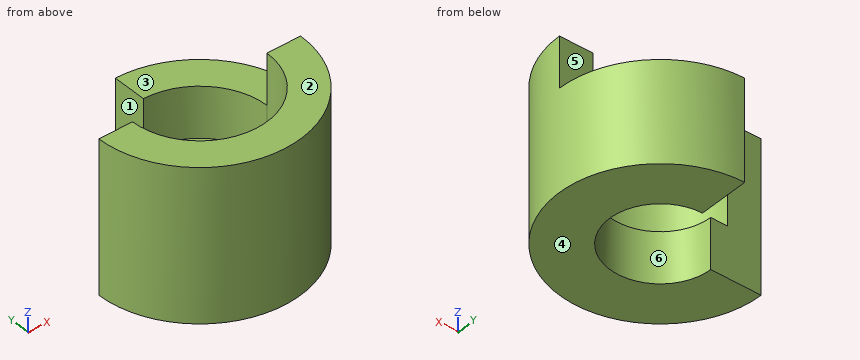
```python
from build123d import *

# Parameters (mm, degrees)
BOSS_EXTRUDE1_DEPTH = 9
SKETCH2_W           = 6
SKETCH2_H           = 6
CUT_EXTRUDE1_DEPTH  = 3
SKETCH3_R           = 4
CUT_EXTRUDE2_DEPTH  = 6


with BuildPart() as part:
    # Sketch1 → Boss-Extrude1 (new body)
    with BuildSketch(Plane.XY):
        with BuildLine():
            Line((-6, 0), (-3, 0))
            ThreePointArc((-3, 0), (2.121320344, -2.121320344), (0, 3))
            Line((0, 3), (0, 6))
            ThreePointArc((0, 6), (4.242640687, -4.242640687), (-6, 0))
        make_face()
    extrude(amount=BOSS_EXTRUDE1_DEPTH)

    # Sketch2 → Cut-Extrude1 (cut)
    with BuildSketch(Plane.XY.offset(9)):
        with Locations((3, 3)):
            Rectangle(SKETCH2_W, SKETCH2_H)
    extrude(amount=-CUT_EXTRUDE1_DEPTH, mode=Mode.SUBTRACT)

    # Sketch3 → Cut-Extrude2 (cut)
    with BuildSketch(Plane.XY.offset(9)):
        Circle(SKETCH3_R)
    extrude(amount=-CUT_EXTRUDE2_DEPTH, mode=Mode.SUBTRACT)


solid = part.part
```
Work out the finished part from the listing and answer in its coordinate system (mm). Face numbers are marked on the shaded views. A direction names the side the tool comes from. Give positions to 0.01 mm unless a question says otherwise; leave off trailing zeros. Loops run counter-clockwise (first coordinate to the right, second up) from the corner with the lowest first, then second, coordinate; pieces in that order, holes last. Notation, with made-up numbers: (83.25, -22.5) -> (135.25, -22.5) arc R32 cw to (135.25, 14.5) -> close; hole circle Ø9 at (-35, 26). An arc over 180 degrees is marked (long way). Write item = value, one per line. Start each with the question number.
(1) Which of the six approach directions +Z, -Z, +X, -X, +Y, -Y give full straight-line access (tool end or side, diameter ignored) to the marked faces 1, 2 and 3?
(2) Find section B-B on z = 5. Give the vertices of the cut face in (x, y), and give its area (3 significant figures).
(3) Find section A-A on y = -0.5. Give the vertices of the cut face in (x, z).
(4) Find section C-C on x = -1.5. Give the vertices of the cut face in (y, z), and give its area (3 significant figures).
(5) Find the intervals of material crossed by probe 1 along Z at (x, y) = (3.75, -0.5); probe 2 along X at (y, z) = (-2.75, 6.75); probe 3 along Z at (x, y) = (4, 1.5), in increasing order. Write a range as from..to.
(6) Given pin 1 Ø3.5 at (y, z) = (5, 4) entering from -X; pin 2 Ø1.8 at (x, y) = (1.5, 3.5) entering from +Z; pin 3 Ø1 at (x, z) = (4.5, 7.5) entering from +Y, each flat-ended and moving along its own axis, determine where each tip first touches the part or whether it passes through.
(7) The mould has two halves that part along Y. Classify the marked faces 4, 5 and 6: +Y half, -Y half, draft (parallel to the pull), parting line (faces both ways), or undercut.
(8) Find section D-D on y = -3.5. Give the vertices of the cut face in (x, z), and give its area (3 significant figures).
From the geometry:
q1.face_1 = +Z, -Z, -X, +Y
q1.face_2 = +Z, +X, -X, +Y, -Y
q1.face_3 = +Z, +X, -X, +Y
q2.outline = (-6, 0) arc R6 ccw (long way) to (0, 6) -> (0, 4) arc R4 cw (long way) to (-4, 0) -> close
q2.area = 47.1 mm^2
q3.outline = (-5.98, 0) -> (-2.96, 0) -> (-2.96, 3) -> (-3.97, 3) -> (-3.97, 9) -> (-5.98, 9) -> close; (2.96, 0) -> (5.98, 0) -> (5.98, 9) -> (3.97, 9) -> (3.97, 3) -> (2.96, 3) -> close
q4.outline = (-5.81, 0) -> (-2.6, 0) -> (-2.6, 3) -> (-3.71, 3) -> (-3.71, 9) -> (-5.81, 9) -> close
q4.area = 22.2 mm^2
q5.probe_1 = 0..3
q5.probe_2 = -5.33..-2.9, 2.9..5.33
q5.probe_3 = 0..6
q6.pin_1 = 0
q6.pin_2 = 6
q6.pin_3 = 0
q7.face_4 = draft
q7.face_5 = +Y half
q7.face_6 = undercut
q8.outline = (-4.87, 0) -> (4.87, 0) -> (4.87, 9) -> (1.94, 9) -> (1.94, 3) -> (-1.94, 3) -> (-1.94, 9) -> (-4.87, 9) -> close
q8.area = 64.5 mm^2
